Read the model definition and answer for the solid it produces. Units are mm, in the model's axes. Face numbers are marked on the shaded views. A direction names the side the tool comes from. Coordinates: 2 decimals unless noted, no trailing zeros. Loops run counter-clockwise (first coordinate to the right, second up) from the corner with the lowest first, then second, coordinate; pieces in that order, holes last. Notation, with made-up numbers: M 29.25,-3 L 47.25,-3 A16 cw 47.25,23 Z; hole C 52,-33.75 d5. An arc over 180 degrees is marked long. Use one line per item in the form item = value. Start each with the question number.
1. A tool of negligible diameter and unlimited length cuts with its end or side. For the marked faces 1, 2, 3, 4 and 5, from which of +Z, -Z, +X, -X, +Y, -Y can it reach the whole face along a straight path? Write none if from no direction.
2. For a pull along Z with two mould halves and no side action, classify the marked faces 6, 7, 8 and 9 as released by +Z, released by -Z, zero draft, split by the parting line, or undercut.
3. The part is cut by section C-C (x = 32). Give the vertices of the cut face in (y, z), plus the area to 3 significant figures.
4. Find the intervals of material crossed by probe 1 along Z at (x, y) = (0, -9.25); probe 2 along X at (y, z) = (-22.5, -37.5); probe 3 along Z at (x, y) = (-32, -11.5), in increasing order. Write a range as [from, to].
5. The part is cut by section B-B (x = 0). Give the vertices of the cut face in (y, z), plus the area to 3 significant figures.
6. Flat-ended cylindrical pins translate along their axes: pin 1 (10 mm diameter, centred on x = 23.5, y = -12, fed in from -Z); pin 2 (8 mm diameter, centred on x = 8.5, y = -18.5, fed in from +Z); pin 3 (5 mm diameter, centred on y = -9.5, z = -9, fed in from -X). Find the tip coordinate at first contact, or state that the pin passes through.
7. The part is cut by section A-A (z = 0). Give the vertices of the cut face in (x, y).
8. The part is cut by section D-D (z = -32). Give the vertices of the cut face in (x, y), plus the area to 3 significant figures.
from build123d import *

# Parameters (mm, degrees)
F0_R     = 17.907
F1_DEPTH = 25.4


with BuildPart() as f1:
    # F0 (on Front) → F1 (new body)
    with BuildSketch(Plane.XZ):
        with BuildLine():
            Line((42.05466, 3.034541), (37.142847, 3.812496))
            ThreePointArc((37.142847, 3.812496), (36.770752, 6.483676), (36.20681, 9.121028))
            Line((36.20681, 9.121028), (40.556328, 11.532005))
            ThreePointArc((40.556328, 11.532005), (39.6212, 14.420937), (38.48058, 17.235077))
            Line((38.48058, 17.235077), (33.598909, 16.286176))
            ThreePointArc((33.598909, 16.286176), (32.335657, 18.669), (30.903697, 20.954421))
            Line((30.903697, 20.954421), (34.166304, 24.707621))
            Line((34.166304, 24.707621), (30.265173, 29.356808))
            Line((30.265173, 29.356808), (26.002447, 26.795504))
            ThreePointArc((26.002447, 26.795504), (24.000404, 28.602567), (21.873142, 30.260401))
            Line((21.873142, 30.260401), (23.65532, 34.903134))
            ThreePointArc((23.65532, 34.903134), (21.082, 36.515095), (18.39934, 37.937675))
            Line((18.39934, 37.937675), (15.269705, 34.072897))
            ThreePointArc((15.269705, 34.072897), (12.770348, 35.086243), (10.204363, 35.916531))
            Line((10.204363, 35.916531), (10.291155, 40.888813))
            Line((10.291155, 40.888813), (4.314275, 41.942698))
            Line((4.314275, 41.942698), (2.695212, 37.240597))
            ThreePointArc((2.695212, 37.240597), (0, 37.338), (-2.695212, 37.240597))
            Line((-2.695212, 37.240597), (-4.314275, 41.942698))
            ThreePointArc((-4.314275, 41.942698), (-7.321702, 41.523434), (-10.291155, 40.888813))
            Line((-10.291155, 40.888813), (-10.204363, 35.916531))
            ThreePointArc((-10.204363, 35.916531), (-12.770348, 35.086243), (-15.269705, 34.072897))
            Line((-15.269705, 34.072897), (-18.39934, 37.937675))
            Line((-18.39934, 37.937675), (-23.65532, 34.903134))
            Line((-23.65532, 34.903134), (-21.873142, 30.260401))
            ThreePointArc((-21.873142, 30.260401), (-24.000404, 28.602567), (-26.002447, 26.795504))
            Line((-26.002447, 26.795504), (-30.265173, 29.356808))
            ThreePointArc((-30.265173, 29.356808), (-32.299498, 27.102497), (-34.166304, 24.707621))
            Line((-34.166304, 24.707621), (-30.903697, 20.954421))
            ThreePointArc((-30.903697, 20.954421), (-32.335657, 18.669), (-33.598909, 16.286176))
            Line((-33.598909, 16.286176), (-38.48058, 17.235077))
            Line((-38.48058, 17.235077), (-40.556328, 11.532005))
            Line((-40.556328, 11.532005), (-36.20681, 9.121028))
            ThreePointArc((-36.20681, 9.121028), (-36.770752, 6.483676), (-37.142847, 3.812496))
            Line((-37.142847, 3.812496), (-42.05466, 3.034541))
            ThreePointArc((-42.05466, 3.034541), (-42.164, 0), (-42.05466, -3.034541))
            Line((-42.05466, -3.034541), (-37.142847, -3.812496))
            ThreePointArc((-37.142847, -3.812496), (-36.770752, -6.483676), (-36.20681, -9.121028))
            Line((-36.20681, -9.121028), (-40.556328, -11.532005))
            Line((-40.556328, -11.532005), (-38.48058, -17.235077))
            Line((-38.48058, -17.235077), (-33.598909, -16.286176))
            ThreePointArc((-33.598909, -16.286176), (-32.335657, -18.669), (-30.903697, -20.954421))
            Line((-30.903697, -20.954421), (-34.166304, -24.707621))
            ThreePointArc((-34.166304, -24.707621), (-32.299498, -27.102497), (-30.265173, -29.356808))
            Line((-30.265173, -29.356808), (-26.002447, -26.795504))
            ThreePointArc((-26.002447, -26.795504), (-24.000404, -28.602567), (-21.873142, -30.260401))
            Line((-21.873142, -30.260401), (-23.65532, -34.903134))
            Line((-23.65532, -34.903134), (-18.39934, -37.937675))
            Line((-18.39934, -37.937675), (-15.269705, -34.072897))
            ThreePointArc((-15.269705, -34.072897), (-12.770348, -35.086243), (-10.204363, -35.916531))
            Line((-10.204363, -35.916531), (-10.291155, -40.888813))
            ThreePointArc((-10.291155, -40.888813), (-7.321702, -41.523434), (-4.314275, -41.942698))
            Line((-4.314275, -41.942698), (-2.695212, -37.240597))
            ThreePointArc((-2.695212, -37.240597), (0, -37.338), (2.695212, -37.240597))
            Line((2.695212, -37.240597), (4.314275, -41.942698))
            Line((4.314275, -41.942698), (10.291155, -40.888813))
            Line((10.291155, -40.888813), (10.204363, -35.916531))
            ThreePointArc((10.204363, -35.916531), (12.770348, -35.086243), (15.269705, -34.072897))
            Line((15.269705, -34.072897), (18.39934, -37.937675))
            ThreePointArc((18.39934, -37.937675), (21.082, -36.515095), (23.65532, -34.903134))
            Line((23.65532, -34.903134), (21.873142, -30.260401))
            ThreePointArc((21.873142, -30.260401), (24.000404, -28.602567), (26.002447, -26.795504))
            Line((26.002447, -26.795504), (30.265173, -29.356808))
            Line((30.265173, -29.356808), (34.166304, -24.707621))
            Line((34.166304, -24.707621), (30.903697, -20.954421))
            ThreePointArc((30.903697, -20.954421), (32.335657, -18.669), (33.598909, -16.286176))
            Line((33.598909, -16.286176), (38.48058, -17.235077))
            ThreePointArc((38.48058, -17.235077), (39.6212, -14.420937), (40.556328, -11.532005))
            Line((40.556328, -11.532005), (36.20681, -9.121028))
            ThreePointArc((36.20681, -9.121028), (36.770752, -6.483676), (37.142847, -3.812496))
            Line((37.142847, -3.812496), (42.05466, -3.034541))
            Line((42.05466, -3.034541), (42.05466, 3.034541))
        make_face()
        Circle(F0_R, mode=Mode.SUBTRACT)
    extrude(amount=F1_DEPTH)


solid = f1.part
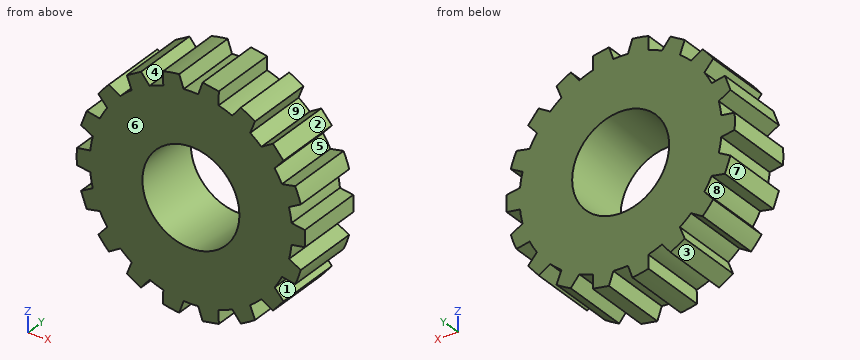
Computed values:
q1.face_1 = +X, +Y, -Y
q1.face_2 = +Z, +X, +Y, -Y
q1.face_3 = -Z, -X, +Y, -Y
q1.face_4 = +Z, +Y, -Y
q1.face_5 = +Y, -Y
q2.face_6 = zero draft
q2.face_7 = released by -Z
q2.face_8 = undercut
q2.face_9 = undercut
q3.outline = M -25.4,-27.29 L 0,-27.29 L 0,-22.22 L -25.4,-22.22 Z; M -25.4,-19.24 L 0,-19.24 L 0,19.24 L -25.4,19.24 Z; M -25.4,22.22 L 0,22.22 L 0,27.29 L -25.4,27.29 Z
q3.area = 1,240 mm²
q4.probe_1 = [-37.34, -17.91], [17.91, 37.34]
q4.probe_2 = [-19.16, -18.04], [-10.23, -2.78], [2.78, 10.23], [18.04, 19.28]
q4.probe_3 = [-27.46, -22.22], [-19.24, 19.24], [22.22, 27.46]
q5.outline = M -25.4,-37.34 L 0,-37.34 L 0,-17.91 L -25.4,-17.91 Z; M -25.4,17.91 L 0,17.91 L 0,37.34 L -25.4,37.34 Z
q5.area = 987 mm²
q6.pin_1 = -37.89
q6.pin_2 = 41.91
q6.pin_3 = -40.5
q7.outline = M -42.16,-25.4 L -17.91,-25.4 L -17.91,0 L -42.16,0 Z; M 17.91,-25.4 L 42.05,-25.4 L 42.05,0 L 17.91,0 Z
q8.outline = M -22.54,-25.4 L 22.54,-25.4 L 22.54,0 L -22.54,0 Z
q8.area = 1,150 mm²
